Part model, mm, in its own coordinate system. Face numbers are marked on the shaded views. A direction names the side the tool comes from. Round coordinates to 2 decimals unless told otherwise and drop trailing zeros. Write each loop counter-clockwise with the first axis right and the second up, starting at its lowest first coordinate (ties: lowest second). Pieces come first, ordered by that corner, then holes. Notation, with made-up numbers: M 88.5,-23.75 L 123.5,-23.75 A14 ccw 123.5,-16.75 Z; hole C 14,-38.75 d1. An arc over 180 degrees is marked long. One line per question, with ' | ' between items. Start each with the question number.
1) Wall check: probe 1 along Z at (x, y) = (-34, 74); probe 2 along Y at (x, z) = (-33, -6); probe 3 along Y at (x, z) = (-23, -31) (3 decimals). Give the ranges that are in metal, low to high. Write a range as [from, to].
2) Drop flat-ended pins along their axis: pin 1 Ø6 at (y, z) = (69, -27) entering from +X; pin 2 Ø4 at (x, y) = (11, 33) entering from -Z; pin 3 Ø1.5 at (x, z) = (-17, -51) entering from -Y; pin 4 Ø13.5 at (x, y) = (-29.11, 50.95) entering from -Z. Give the stop position or say it passes through.
3) Saw through at A-A (y = 84.5). List the corners of the cut face in (x, z).
4) Tool access for the marked faces 1, 2, 3 and 4: list every direction of +Z, -Z, +X, -X, +Y, -Y with a clear straight run to the whole face (end or side of a thin tool).
5) Saw through at B-B (z = -25.5). List the corners of the cut face in (x, y).
6) Saw through at C-C (x = -39.5). List the corners of the cut face in (y, z), plus the area to 3 significant figures.
7) Mould opens along X. For the marked faces 5, 6 and 7 say: pulls with the +X half, pulls with the -X half, needs draft (parallel to the pull), parting line crosses it, or undercut.
```python
from build123d import *

# Parameters (mm, degrees)
SKETCH3_R           = 17.5
BOSS_EXTRUDE2_DEPTH = 100
SKETCH4_R           = 7.5
CUT_EXTRUDE2_DEPTH  = 100
BOSS_EXTRUDE6_DEPTH = 45
SKETCH18_W          = 14.667250813
SKETCH18_H          = 27.752479941
CUT_EXTRUDE6_DEPTH  = 45
SKETCH19_W          = 15.940771985
SKETCH19_H          = 23.227982035
CUT_EXTRUDE8_DEPTH  = 45
BOSS_EXTRUDE8_DEPTH = 25


with BuildPart() as part:
    # Sketch3 → Boss-Extrude2 (new body)
    with BuildSketch(Plane.XY):
        with Locations((-29.114826613, 50.947684889)):
            Circle(SKETCH3_R)
    extrude(amount=-BOSS_EXTRUDE2_DEPTH)

    # Sketch4 → Cut-Extrude2 (cut)
    with BuildSketch(Plane.XY):
        with Locations((-29.114826613, 50.947684889)):
            Circle(SKETCH4_R)
    extrude(amount=-CUT_EXTRUDE2_DEPTH, mode=Mode.SUBTRACT)

    # Sketch16 → Boss-Extrude6 (add)
    with BuildSketch(Plane.XY):
        Polygon((-11.698148649, 52.653360332), (15.559104196, 42.84895981), (15.359838121, 28.805969908), (-15.52924146, 39.916734066), align=None)
    extrude(amount=-BOSS_EXTRUDE6_DEPTH)

    # Sketch18 → Cut-Extrude6 (cut)
    with BuildSketch(Plane(origin=(15.429488543, 42.895582402, 0), x_dir=(0.940977711, -0.338468532, 0), z_dir=(0.338468532, 0.940977711, 0))):
        with Locations((-21.495577319, 13.876239971)):
            Rectangle(SKETCH18_W, SKETCH18_H)
    extrude(amount=-CUT_EXTRUDE6_DEPTH, mode=Mode.SUBTRACT)

    # Sketch19 → Cut-Extrude8 (cut)
    with BuildSketch(Plane(origin=(15.429488543, 42.895582402, 0), x_dir=(0.940977711, -0.338468532, 0), z_dir=(0.338468532, 0.940977711, 0))):
        with Locations((4.556401634, 22.58985628)):
            Rectangle(SKETCH19_W, SKETCH19_H)
    extrude(amount=-CUT_EXTRUDE8_DEPTH, mode=Mode.SUBTRACT)

    # Sketch20 → Boss-Extrude8 (add)
    with BuildSketch(Plane(origin=(0, 0, -100), x_dir=(-1, 0, 0), z_dir=(0, 0, -1))):
        with BuildLine():
            ThreePointArc((15.84180119, 92.226602563), (30.129018278, 75.909507637), (46.446113204, 90.196724725))
            Line((46.446113204, 90.196724725), (50.037435532, 90.196724725))
            ThreePointArc((50.037435532, 90.196724725), (30.003778847, 72.192945878), (12, 92.226602563))
            Line((12, 92.226602563), (15.84180119, 92.226602563))
        make_face()
        with BuildLine():
            ThreePointArc((36.589403128, 72.998778341), (30.377850806, 72.176669134), (24.235659001, 73.414702098))
            Line((24.235659001, 73.414702098), (24.235659001, 67.753746992))
            ThreePointArc((24.235659001, 67.753746992), (30.50242594, 68.392585809), (36.589403128, 66.771107588))
            Line((36.589403128, 66.771107588), (36.589403128, 72.998778341))
        make_face()
    extrude(amount=-BOSS_EXTRUDE8_DEPTH)


solid = part.part
```
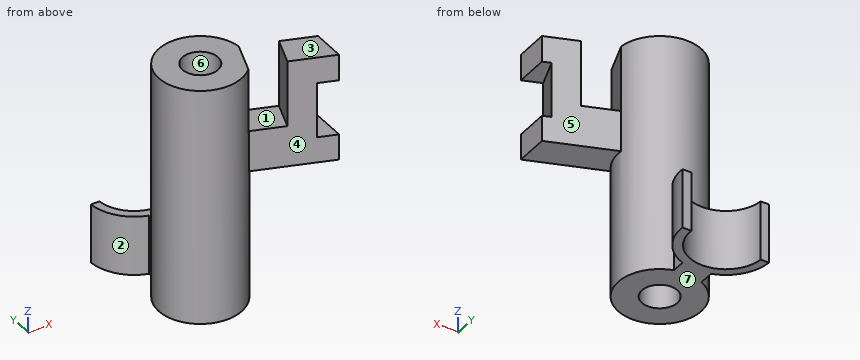
Answer key:
1) probe 1: z = [-100, -75] | probe 2: y = [33.88, 44.53], [57.36, 68.01] | probe 3: y = [34.551, 46.605], [55.29, 67.345]
2) pin 1: stops at x = -20.19 | pin 2: stops at z = -45 | pin 3: stops at y = 37.64 | pin 4: passes through
3) outline: M -48.84,-100 L -44.93,-100 L -44.93,-75 L -48.84,-75 Z; M -17.35,-100 L -13.19,-100 L -13.19,-75 L -17.35,-75 Z
4) face 1: +Z | face 2: +Z, -Z, -X | face 3: +Z, +X, -X, +Y, -Y | face 4: +Z, -Z, -Y
5) outline: M -16.78,38.54 L -11.7,52.65 A17.5 ccw long Z; M -2.39,35.19 L 7.72,31.55 L 12.22,44.05 L 2.1,47.69 Z; hole C -29.11,50.95 d15
6) outline: M 36.86,-100 L 65.03,-100 L 65.03,0 L 36.86,0 Z; M 74.16,-100 L 78.35,-100 L 78.35,-75 L 74.16,-75 Z | area: 2,920 mm2
7) face 5: pulls with the +X half | face 6: undercut | face 7: needs draft
